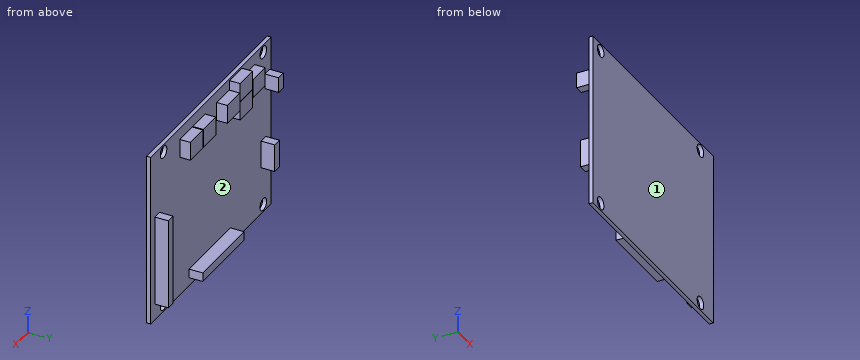
from build123d import *

# Parameters (mm, degrees)
SKETCH1_W             = 92
SKETCH1_H             = 70.1
SKETCH1_R             = 2.5
Y_PCB_EXTR_DEPTH      = 1.6
SKETCH2_W             = 31.55
SKETCH2_H             = 3.6
SKETCH2_W_2           = 3.6
SKETCH2_H_2           = 11.2
SKETCH2_H_3           = 6.15
SKETCH2_H_4           = 36.6
Y_HEADERS_EXTR_DEPTH  = 5.54
SKETCH3_W             = 9.5
SKETCH3_H             = 7.5
Y_SWITCHES_EXTR_DEPTH = 4.3


with BuildPart() as part:
    # Sketch1 → Y+ PCB extr (new body)
    with BuildSketch(Plane(origin=(0, 0, 0), x_dir=(1, 0, 0), z_dir=(0, 1, 0))):
        with Locations((46, 35.05)):
            Rectangle(SKETCH1_W, SKETCH1_H)
        with Locations(Location((5.92, 3.07, 0), (0, 0, 270))):
            Circle(SKETCH1_R, mode=Mode.SUBTRACT)
        with Locations(Location((82.16, 3.11, 0), (0, 0, 270))):
            Circle(SKETCH1_R, mode=Mode.SUBTRACT)
        with Locations(Location((82.16, 67.05, 0), (0, 0, 270))):
            Circle(SKETCH1_R, mode=Mode.SUBTRACT)
        with Locations(Location((5.92, 67.1, 0), (0, 0, 270))):
            Circle(SKETCH1_R, mode=Mode.SUBTRACT)
    extrude(amount=Y_PCB_EXTR_DEPTH)

    # Sketch2 → Y+ headers extr (add)
    with BuildSketch(Plane(origin=(0, 1.6, 0), x_dir=(1, 0, 0), z_dir=(0, 1, 0))):
        with Locations((46.775, 65.02)):
            Rectangle(SKETCH2_W, SKETCH2_H)
        with Locations((5.92, 45.09)):
            Rectangle(SKETCH2_W_2, SKETCH2_H_2)
        with Locations((2.92, 15.995)):
            Rectangle(SKETCH2_W_2, SKETCH2_H_3)
        with Locations((87.08, 45.11)):
            Rectangle(SKETCH2_W_2, SKETCH2_H_4)
    extrude(amount=Y_HEADERS_EXTR_DEPTH)

    # Sketch3 → Y+ switches extr (add)
    with BuildSketch(Plane(origin=(0, 1.6, 0), x_dir=(1, 0, 0), z_dir=(0, 1, 0))):
        with Locations((17.32, 8.42)):
            Rectangle(SKETCH3_W, SKETCH3_H)
        with Locations((26.98, 4.61)):
            Rectangle(SKETCH3_W, SKETCH3_H)
        with Locations((26.98, 12.41)):
            Rectangle(SKETCH3_W, SKETCH3_H)
        with Locations((36.78, 8.42)):
            Rectangle(SKETCH3_W, SKETCH3_H)
        with Locations((55.12, 8.42)):
            Rectangle(SKETCH3_W, SKETCH3_H)
        with Locations((65.02, 8.42)):
            Rectangle(SKETCH3_W, SKETCH3_H)
    extrude(amount=Y_SWITCHES_EXTR_DEPTH)


solid = part.part
Here's how the part is built. I have some questions about the finished solid (model axes, mm). Face numbers are marked on the shaded views. Coordinates: 2 decimals unless noted, no trailing zeros. Loops run counter-clockwise (first coordinate to the right, second up) from the corner with the lowest first, then second, coordinate; pieces in that order, holes last.
1. I need wall thicknesses on L1, parallel to X at y = 0.7, z = -67.1; L2, parallel to X at y = 1, z = -66.5; L3, parallel to X at y = 5.5, z = -14. Which ranges of each line are inside material? Lowest first, please.
2. If we mould it in two halves opening along Z, with no side actions, what happens to the marked faces 1 and 2? For each: pulls with the +Z half, pulls with the -Z half, needs draft (parallel to the pull), parting line crosses it, or undercut.
3. Imagine slicing it at A-A, the plane x = 5.92. Please give me the cut outline in (y, z).
4. Imagine slicing it at B-B, the plane x = 45. Please give me the cut outline in (y, z).
5. For P1, Ø1, axis at x = 21, y = 4.5, coming from the -Z side; P2, Ø3.5, axis at x = 62.5, y = 4.5, coming from the -Z side; P3, Ø1.8, axis at x = 5, y = 5, coming from the -Z side, each with a flat end and sliding along its axis, tell me the tip position at first contact or that it passes through.
6. Imagine slicing it at D-D, the plane z = -3.11. Please give me the cut outline in (x, y), and give its area (3 significant figures).
7. Imagine slicing it at C-C, the plane z = -53. Please give me the cut outline in (x, y).
Taken from the geometry:
1. L1: x = 0 to 3.42, 8.42 to 79.66, 84.66 to 92
1. L2: x = 0 to 3.49, 8.35 to 79.72, 84.6 to 92
1. L3: x = 1.12 to 4.72, 22.23 to 31.73
2. face 1: needs draft
2. face 2: undercut
3. outline: (0, -70.1) - (1.6, -70.1) - (1.6, -69.6) - (0, -69.6) - close; (0, -64.6) - (1.6, -64.6) - (1.6, -50.69) - (7.14, -50.69) - (7.14, -39.49) - (1.6, -39.49) - (1.6, -5.57) - (0, -5.57) - close; (0, -0.57) - (1.6, -0.57) - (1.6, 0) - (0, 0) - close
4. outline: (0, -70.1) - (1.6, -70.1) - (1.6, -66.82) - (7.14, -66.82) - (7.14, -63.22) - (1.6, -63.22) - (1.6, 0) - (0, 0) - close
5. P1: stops at z = -12.17
5. P2: stops at z = -66.82
5. P3: stops at z = -50.69
6. outline: (0, 0) - (3.42, 0) - (3.42, 1.6) - (0, 1.6) - close; (8.42, 0) - (79.66, 0) - (79.66, 1.6) - (31.73, 1.6) - (31.73, 5.9) - (22.23, 5.9) - (22.23, 1.6) - (8.42, 1.6) - close; (84.66, 0) - (92, 0) - (92, 1.6) - (84.66, 1.6) - close
6. area: 172 mm2
7. outline: (0, 0) - (92, 0) - (92, 1.6) - (88.88, 1.6) - (88.88, 7.14) - (85.28, 7.14) - (85.28, 1.6) - (0, 1.6) - close
